Verification items for this drawing (mm, ordinates from the low corner). A direction names the side the tool comes from. Give positions to 0.01 mm unless a question says otherwise; leave off trailing zeros. Order: outer loops, then holes, each group sorted by start corner. A loop starts at its lowest first (then second) coordinate and runs counter-clockwise, first axis right, second up.
(1) Gauge pin test, flat ends, axial feed: pin 1 (4 mm diameter, centred on y = 53.5, z = 17.5, fed in from +X); pin 2 (5 mm diameter, centred on x = 27.5, z = 47, fed in from +Y); pin 3 (12 mm diameter, centred on y = 56, z = 26.5, fed in from +X) (1 decimal); pin 4 (10 mm diameter, centred on x = 33.5, y = 40.5, fed in from +Z). Record the tip position at first contact, or that the pin passes through.
(2) Sectioned sample at A-A on z = 30. Record the cut outline in (x, y) (1 decimal), plus the area to 3 significant figures.
(3) Access from +Z, -Z, +X, -X, +Y, -Y to the whole of each face (thin tool, end or side, straight path). Record for the marked faces 1 and 2.
(4) Sectioned sample at C-C on x = 24. Record the cut outline in (y, z), plus the area to 3 significant figures.
(5) Sectioned sample at B-B on x = 41.5. Record the cut outline in (y, z).
(6) Scan lines: L1, parallel to Y at x = 11, z = 68; L2, parallel to Y at x = 49.5, z = 81; L3, parallel to X at y = 29, z = 30 (1 decimal). Record each from-to range of solid material in increasing order.
(7) Sectioned sample at D-D on y = 46. Record the cut outline in (x, z), plus the area to 3 significant figures.
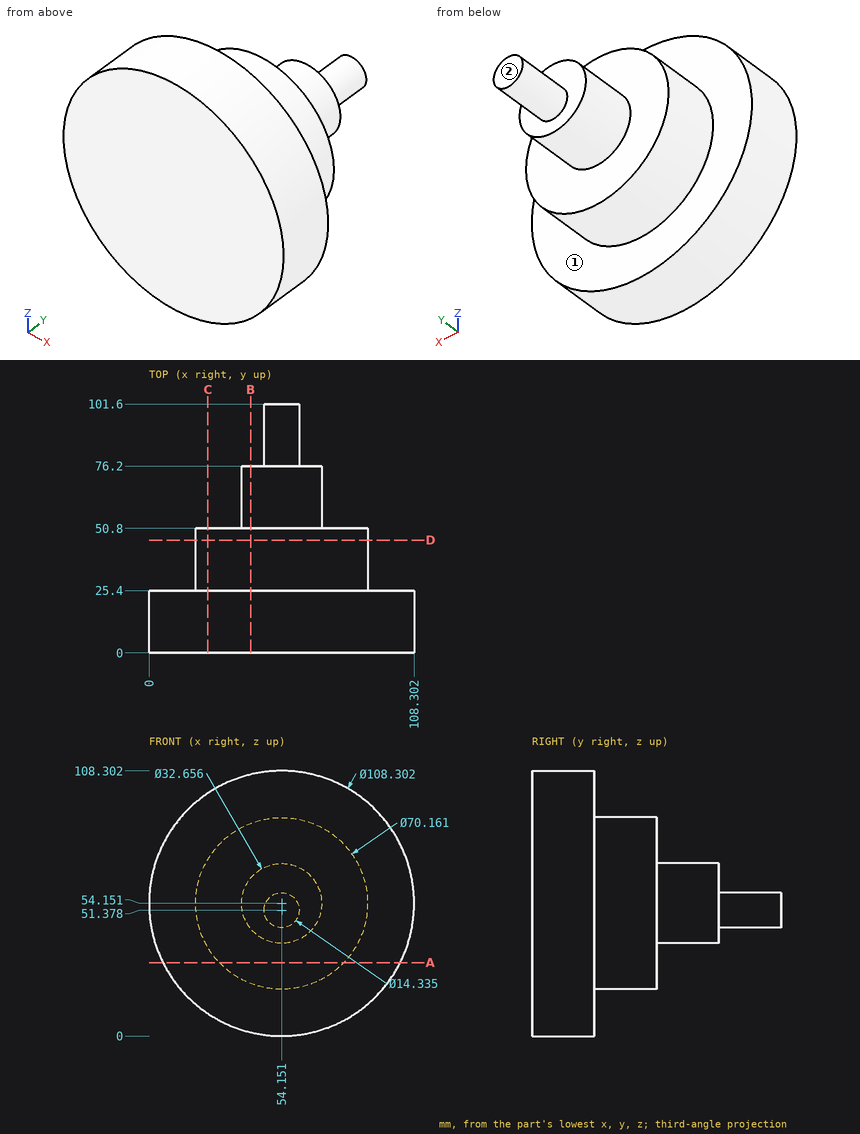
Ans:
1. pin 1: passes through
1. pin 2: stops at y = 50.8
1. pin 3: stops at x = 79.1
1. pin 4: stops at z = 85.55
2. outline: (5.7, 0) - (102.6, 0) - (102.6, 25.4) - (79.6, 25.4) - (79.6, 50.8) - (28.7, 50.8) - (28.7, 25.4) - (5.7, 25.4) - close
2. area: 3,750 mm2
3. face 1: +Y
3. face 2: +Z, -Z, +X, -X, +Y
4. outline: (0, 9.17) - (25.4, 9.17) - (25.4, 36.22) - (50.8, 36.22) - (50.8, 72.08) - (25.4, 72.08) - (25.4, 99.13) - (0, 99.13) - close
4. area: 3,200 mm2
5. outline: (0, 1.5) - (25.4, 1.5) - (25.4, 21.43) - (50.8, 21.43) - (50.8, 43.83) - (76.2, 43.83) - (76.2, 64.47) - (50.8, 64.47) - (50.8, 86.87) - (25.4, 86.87) - (25.4, 106.8) - (0, 106.8) - close
6. L1: y = 0 to 25.4
6. L2: y = 0 to 50.8
6. L3: x = 28.7 to 79.6
7. outline: circle Ø70.16 at (54.15, 54.15)
7. area: 3,870 mm2
